Model file for the job. Use its own axes, mm. A direction names the side the tool comes from. Round coordinates to 2 decimals unless told otherwise and drop trailing zeros. Order: outer loops, then holes, each group sorted by start corner. A loop starts at its lowest first (then second) coordinate and runs counter-clockwise, first axis right, second up. Notation, with made-up numbers: (75.25, 27.25) - (119.25, 27.25) arc R20 ccw to (119.25, 63.25) - close; hole circle Ø3 at (-6, 49.25). An arc over 180 degrees is marked (long way). Answer as CSV lines item,"result". Start each with the question number.
1. 3-axis set-ups, long thin cutter, end or side, ignore diameter. For faces 1 (the face through (0, 0, -1.905)), 2 (the face through (26.62, -0.08, 3.81)), 3 (the face through (0.28, -0.08, 2.41)), 4 (the face through (-20.32, 0, 0)): which of +Z, -Z, +X, -X, +Y, -Y reach the whole face in a straight line?
2. Pin check, flat tips, straight feed: pin 1 Ø6 at (x, y) = (4.5, 2.5) entering from -Z (3 decimals); pin 2 Ø1 at (x, z) = (24, -3.5) entering from +Y; pin 3 Ø7.5 at (y, z) = (-0.5, -2) entering from +X. Stop position of each tip, or through.
3. Band-saw the part on C-C on x = 22. List the corners of the cut face in (y, z).
4. Band-saw the part on B-B on y = 0.5. List the corners of the cut face in (x, z) (3 decimals).
5. Wall check: line 1 along X through (y, z) = (-1, 1.75); line 2 along X through (y, z) = (1.75, -5.75); line 3 along Z through (x, y) = (-17, 0) (3 decimals). Give the ranges that are in metal, low to high. Write a range as [from, to].
6. Band-saw the part on D-D on z = 4.75. List the corners of the cut face in (x, y), then the cut area to 3 significant figures.
7. Band-saw the part on A-A on z = 0. List the corners of the cut face in (x, y).
```python
from build123d import *

# Parameters (mm, degrees)
BOSS_EXTRUDE1_DEPTH = 20.32
SKETCH2_R           = 7.62
BOSS_EXTRUDE2_DEPTH = 2.54
SKETCH3_R           = 1.905
BOSS_EXTRUDE3_DEPTH = 7.62


with BuildPart() as part:
    # Sketch1 → Boss-Extrude1 (new, symmetric)
    with BuildSketch(Plane(origin=(0, 0, 0), x_dir=(0, 0, -1), z_dir=(1, 0, 0))):
        with BuildLine():
            Line((1.905, 1.481061781), (1.905, -1.481061781))
            ThreePointArc((1.905, -1.481061781), (-2.413, 0), (1.905, 1.481061781))
        make_face()
    extrude(amount=BOSS_EXTRUDE1_DEPTH, both=True)

    # Sketch2 → Boss-Extrude2 (add)
    with BuildSketch(Plane(origin=(20.32, 0, 0), x_dir=(0, 0, -1), z_dir=(1, 0, 0))):
        Circle(SKETCH2_R)
    extrude(amount=BOSS_EXTRUDE2_DEPTH)

    # Sketch3 → Boss-Extrude3 (add)
    with BuildSketch(Plane(origin=(22.86, 0, 0), x_dir=(0, 0, -1), z_dir=(1, 0, 0))):
        with Locations(Location((-5.715, 0, 0), (0, 0, 179.999322122))):
            Circle(SKETCH3_R)
    extrude(amount=BOSS_EXTRUDE3_DEPTH)


solid = part.part
```
Reply:
1,face 1,"-Z, -X, +Y, -Y"
1,face 2,"+X"
1,face 3,"-X"
1,face 4,"+Z, -Z, -X, +Y, -Y"
2,pin 1,"stops at z = -1.905"
2,pin 2,"passes through"
2,pin 3,"stops at x = 22.86"
3,outline,"circle Ø15.24 at (0, 0)"
4,outline,"(-20.32, -1.905) - (20.32, -1.905) - (20.32, -7.604) - (22.86, -7.604) - (22.86, 3.877) - (30.48, 3.877) - (30.48, 7.553) - (22.86, 7.553) - (22.86, 7.604) - (20.32, 7.604) - (20.32, 2.361) - (-20.32, 2.361) - close"
5,line 1,"x = [-20.32, 22.86]"
5,line 2,"x = [20.32, 22.86]"
5,line 3,"z = [-1.905, 2.413]"
6,outline,"(20.32, -5.96) - (22.86, -5.96) - (22.86, -1.64) - (30.48, -1.64) - (30.48, 1.64) - (22.86, 1.64) - (22.86, 5.96) - (20.32, 5.96) - close"
6,area,"55.3 mm2"
7,outline,"(-20.32, -2.41) - (20.32, -2.41) - (20.32, -7.62) - (22.86, -7.62) - (22.86, 7.62) - (20.32, 7.62) - (20.32, 2.41) - (-20.32, 2.41) - close"
